```python
from build123d import *

# Parameters (mm, degrees)
F1_DEPTH = 1.27
F2_R     = 9.2075
F2_R_2   = 4.7625
F3_DEPTH = 25.4
F4_W     = 16.7551115155
F4_H     = 1.524
F5_DEPTH = 25.4
F6_R     = 2.53999


# Not quite as in the source:
# - a fillet or chamfer is up to 0.001 mm smaller than in the source, because OpenCascade refuses the exact size


with BuildPart() as f1:
    # F0 (on Top) → F1 (new body, symmetric)
    with BuildSketch(Plane.XY):
        with BuildLine():
            ThreePointArc((-6.7098333333, -7.2008987556), (-5.2579227906, -3.7297804895), (-4.7625, 0))
            ThreePointArc((-4.7625, 0), (-5.2579227906, 3.7297804895), (-6.7098333333, 7.2008987556))
            ThreePointArc((-6.7098333333, 7.2008987556), (-9.8425, 0), (-6.7098333333, -7.2008987556))
        make_face()
        with BuildLine():
            ThreePointArc((-6.7098333333, 7.2008987556), (-5.2579227906, 3.7297804895), (-4.7625, 0))
            ThreePointArc((-4.7625, 0), (-5.2579227906, -3.7297804895), (-6.7098333333, -7.2008987556))
            ThreePointArc((-6.7098333333, -7.2008987556), (0, -9.8425), (6.7098333333, -7.2008987556))
            ThreePointArc((6.7098333333, -7.2008987556), (4.7625, 0), (6.7098333333, 7.2008987556))
            ThreePointArc((6.7098333333, 7.2008987556), (0, 9.8425), (-6.7098333333, 7.2008987556))
        make_face()
        with BuildLine():
            ThreePointArc((-6.7098333333, -7.2008987556), (-9.8425, 0), (-6.7098333333, 7.2008987556))
            ThreePointArc((-6.7098333333, 7.2008987556), (-33.3375, 0), (-6.7098333333, -7.2008987556))
        make_face()
        with BuildLine():
            ThreePointArc((9.8425, 0), (9.0254180189, 3.9264024034), (6.7098333333, 7.2008987556))
            ThreePointArc((6.7098333333, 7.2008987556), (4.7625, 0), (6.7098333333, -7.2008987556))
            ThreePointArc((6.7098333333, -7.2008987556), (9.0254180189, -3.9264024034), (9.8425, 0))
        make_face()
        with BuildLine():
            ThreePointArc((33.3375, 0), (22.7797804895, 13.7920772094), (6.7098333333, 7.2008987556))
            ThreePointArc((6.7098333333, 7.2008987556), (9.0254180189, 3.9264024034), (9.8425, 0))
            ThreePointArc((9.8425, 0), (9.0254180189, -3.9264024034), (6.7098333333, -7.2008987556))
            ThreePointArc((6.7098333333, -7.2008987556), (22.7797804895, -13.7920772094), (33.3375, 0))
        make_face()
    extrude(amount=F1_DEPTH, both=True)

    # F2 (on face) → F3 (cut)
    with BuildSketch(Plane.XY.offset(1.27)):
        with Locations((-19.05, 0)):
            Circle(F2_R)
        with Locations((19.05, 0)):
            Circle(F2_R)
        Circle(F2_R_2)
    extrude(amount=-F3_DEPTH, mode=Mode.SUBTRACT)

    # F4 (on face) → F5 (cut)
    with BuildSketch(Plane.XY.offset(1.27)):
        with Locations((-24.9599442422, 0)):
            Rectangle(F4_W, F4_H)
        with Locations((24.9599442422, 0)):
            Rectangle(F4_W, F4_H)
    extrude(amount=-F5_DEPTH, mode=Mode.SUBTRACT)

    # F6 (radius 2.54 in the source; OpenCascade refuses exactly that, so slightly less here)
    f6_edges = [f1.edges().sort_by_distance(p)[0] for p in [
        (-33.317166, 0.762, 0),
        (-28.225915, 0.762, 0),
        (-28.225915, -0.762, 0),
        (-33.317166, -0.762, 0),
        (28.225915, -0.762, 0),
        (28.225915, 0.762, 0),
        (33.317166, 0.762, 0),
        (33.317166, -0.762, 0),
    ]]
    fillet(f6_edges, radius=F6_R)


solid = f1.part
```
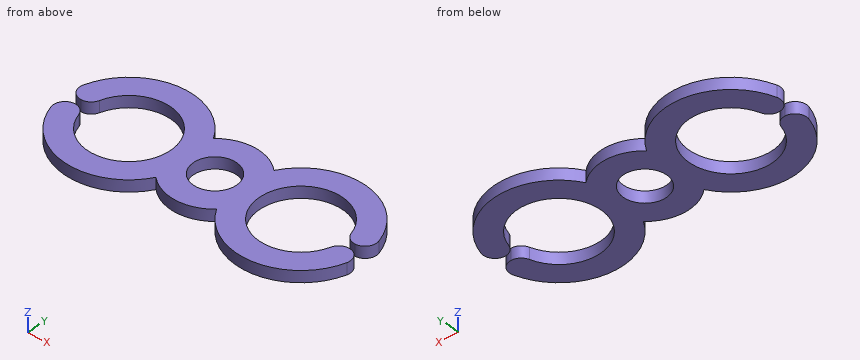
Geometry: final body of the model. Coordinates: model frame, mm. Round coordinates to 2 decimals unless told otherwise and drop trailing zeros. Write each loop counter-clockwise with the first axis right and the second up, starting at its lowest first coordinate (ties: lowest second). Pieces come first, ordered by that corner, then holes. Notation, with made-up numbers: (-37.5, -1.75) -> (-0.5, -1.75) arc R13 ccw to (-0.5, 12.25) -> close; hole circle Ø4 at (14, 17). An arc over 180 degrees is marked (long way). Return JSON: item names as keys, results as strings.
Q1. Ray query, line 1 (Y direction, x = -19.05, z = 0.5); line 2 (X direction, y = -1.75, z = 0.1); line 3 (Y direction, x = 0, z = 0.4). Return the intervals inside material, ascending.
From the geometry:
{"line 1": "-14.29 to -9.21, 9.21 to 14.29", "line 2": "-32.33 to -28.31, -10.01 to -4.43, 4.43 to 10.01, 28.31 to 32.33", "line 3": "-9.84 to -4.76, 4.76 to 9.84"}
Q2. Section A-A on x = -19.05. Return the cut outline in (y, z), and give its area (3 significant figures).
From the geometry:
{"outline": "(-14.29, -1.27) -> (-9.21, -1.27) -> (-9.21, 1.27) -> (-14.29, 1.27) -> close; (9.21, -1.27) -> (14.29, -1.27) -> (14.29, 1.27) -> (9.21, 1.27) -> close", "area": "25.8 mm2"}
Q3. Section D-D on y = -8.25. Return the cut outline in (x, z).
From the geometry:
{"outline": "(-30.71, -1.27) -> (-23.14, -1.27) -> (-23.14, 1.27) -> (-30.71, 1.27) -> close; (-14.96, -1.27) -> (-7.39, -1.27) -> (-7.39, 1.27) -> (-14.96, 1.27) -> close; (-5.37, -1.27) -> (5.37, -1.27) -> (5.37, 1.27) -> (-5.37, 1.27) -> close; (7.39, -1.27) -> (14.96, -1.27) -> (14.96, 1.27) -> (7.39, 1.27) -> close; (23.14, -1.27) -> (30.71, -1.27) -> (30.71, 1.27) -> (23.14, 1.27) -> close"}
Q4. Section C-C on y = 0. Return the cut outline in (x, z).
From the geometry:
{"outline": "(-9.84, -1.27) -> (-4.76, -1.27) -> (-4.76, 1.27) -> (-9.84, 1.27) -> close; (4.76, -1.27) -> (9.84, -1.27) -> (9.84, 1.27) -> (4.76, 1.27) -> close"}
